Read the model definition and answer for the solid it produces. Units are mm, in the model's axes. Coordinates: 2 decimals unless noted, no trailing zeros. Loops run counter-clockwise (first coordinate to the right, second up) from the corner with the lowest first, then second, coordinate; pieces in that order, holes last. Notation, with made-up numbers: M -8,6 L 43,6 A18 cw 43,37 Z; hole C 39.5,-20.5 d10. An arc over 180 degrees is marked long. Use one line per item in the form item = value. Start each with the question number.
1. The part is cut by section A-A (y = 12.5). Give the vertices of the cut face in (x, z).
2. The part is cut by section C-C (y = 7.75). Give the vertices of the cut face in (x, z).
3. Find the intervals of material crossed by probe 1 along Y at (x, z) = (-12.5, 22.05); probe 2 along X at (y, z) = (13.5, 20.4); probe 3 along Y at (x, z) = (-59, 23.8), in increasing order. Write a range as [from, to].
4. For a pull along X with two mould halves and no side action, classify faces 1 (the flat face through (-35, 13, 19)), 2 (the cylindrical face through (-55.592, 13.101, 22.042)), 3 (the cylindrical face through (-0.003, 12.225, 22.042)) as released by +X, released by -X, zero draft, split by the parting line, or undercut.
5. The part is cut by section B-B (z = 19.6). Give the vertices of the cut face in (x, y).
6. The part is cut by section D-D (y = 19.5). Give the vertices of the cut face in (x, z).
7. A flat-ended cylindrical pin translates along its axis: pin 1 (2 mm diameter, centred on y = 17.5, z = 21.5, fed in from -X). Find the tip coordinate at first contact, or state that the pin passes through.
Autodesk Inventor part; units mm, degrees
ref_plane "YZ Plane" through (0, 0, 0) normal (1, 0, 0) x (0, 1, 0)
ref_plane "XZ Plane" through (0, 0, 0) normal (0, 1, 0) x (-1, 0, 0)
ref_plane "XY Plane" through (0, 0, 0) normal (0, 0, 1) x (1, 0, 0)
sketch "Sketch1" plane through (0, 0, 0) normal (0, 0, 1) x (1, 0, 0)
  line L0 (0, 0) -> (-70, 0)
  line L1 (-70, 0) -> (-70, 25)
  line L2 (-70, 25) -> (0, 25)
  line L3 (0, 25) -> (0, 0)
  dimension "d0" = 25
  dimension "d1" = 70
extrude "Extrusion1" add sketch "Sketch1" along normal blind 25
sketch "Sketch3" plane through (0, 0, 25) normal (0, 0, 1) x (1, 0, 0)
  line L0 (0, 0) -> (0, 25)
  line L1 (-70, 0) -> (0, 0)
  circle A0 centre (-12.5, 12.5) radius 12.5
  circle A1 centre (-57.5, 12.5) radius 12.5
  line L2 (-70, 25) -> (-70, 0)
  circle A2 centre (-57.5, 12.5) radius 2
  circle A3 centre (-12.5, 12.5) radius 2
  line L3 (0, 25) -> (-70, 25)
  point P0 (-12.5, 25)
  point P1 (0, 12.5)
  point P2 (-12.5, 0)
  point P3 (-57.5, 25)
  point P4 (-70, 12.5)
  point P5 (-57.5, 0)
extrude "Extrusion2" cut sketch "Sketch3" against normal blind 25 contours L1 A0 L0 | A0 L3 L0 | L1 L2 A1 | A1 L2 L3 | A2 | A3
sketch "Sketch4" plane through (-57.5, 25, 0) normal (0, 1, 0) x (1, 0, 0)
  line L0 (-12.5, 0) -> (-12.5, -25)
  line L1 (57.5, 0) -> (-12.5, 0)
  line L2 (-12.5, 0) -> (-12.5, -19)
  line L3 (-12.5, -19) -> (57.5, -19)
  line L4 (57.5, -19) -> (57.5, 0)
  dimension "d14" = 19
extrude "Extrusion3" cut sketch "Sketch4" against normal blind 100
sketch "Sketch5" plane through (0, 0, 25) normal (0, 0, 1) x (1, 0, 0)
  point P0 (0, 0)
properties part number "Small Rod"
Computed values:
q1.outline = M -70,19 L -59.5,19 L -59.5,25 L -70,25 Z; M -55.5,19 L -14.5,19 L -14.5,25 L -55.5,25 Z; M -10.5,19 L 0,19 L 0,25 L -10.5,25 Z
q2.outline = M -69.06,19 L -0.94,19 L -0.94,25 L -69.06,25 Z
q3.probe_1 = [0, 10.5], [14.5, 25]
q3.probe_2 = [-69.96, -59.23], [-55.77, -14.23], [-10.77, -0.04]
q3.probe_3 = [0.09, 11.18], [13.82, 24.91]
q4.face_1 = zero draft
q4.face_2 = undercut
q4.face_3 = released by +X
q5.outline = M -57.5,0 L -12.5,0 A12.5 ccw -12.5,25 L -57.5,25 A12.5 ccw Z; hole C -57.5,12.5 d4; hole C -12.5,12.5 d4
q6.outline = M -67.86,19 L -2.14,19 L -2.14,25 L -67.86,25 Z
q7.pin_1 = -69.34
